Input: dimensioned drawing with shaded views. Units: mm. Origin: part minimum x, y, z. A direction names the side the tool comes from. Round coordinates to 2 decimals unless told otherwise and drop trailing zeros. Order: outer loops, then holes, each group sorted by start corner. A loop starts at its lowest first (then second) coordinate and runs counter-clockwise, first axis right, second up. Notation, with made-up numbers: M 35,-17 L 50,-17 A22 cw 50,-1 Z; hole C 0.5,67.5 d10. An arc over 180 degrees is marked long. One line per question, with ' | ' between items.
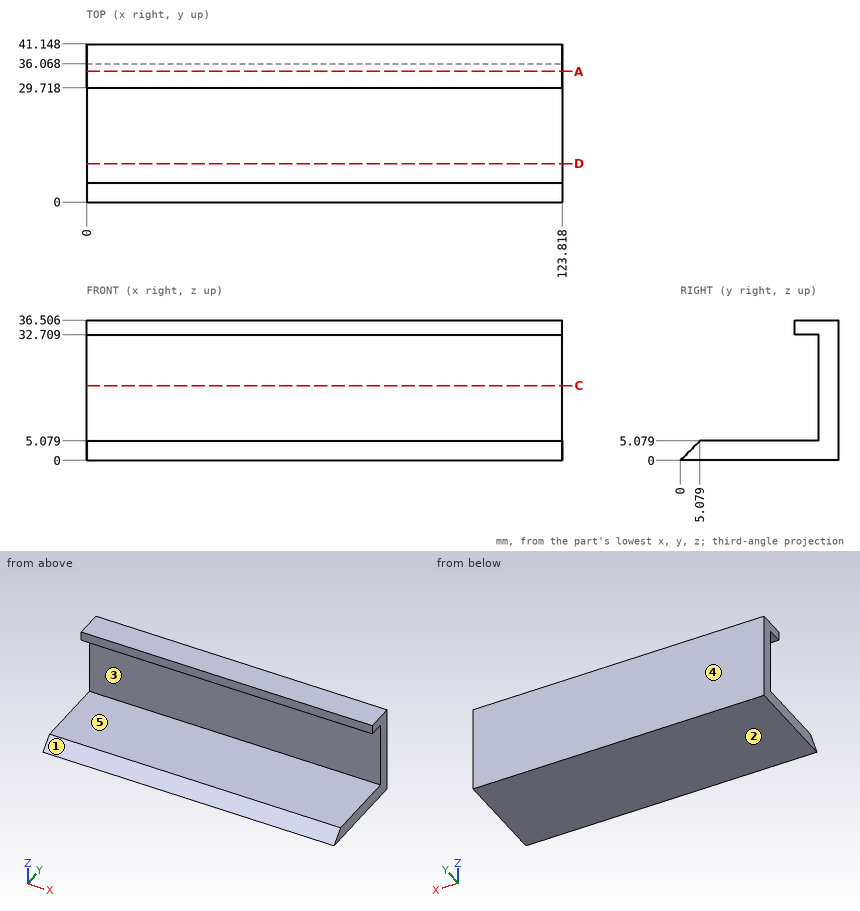
Item 1: Access query for the marked faces 4 and 5. Directions: +Z, -Z, +X, -X, +Y, -Y. A direction counts if a zero-diameter tool reaches every point of the face in a straight line with its end or side. Return the directions, or none.
Report:
face 4: +Z, -Z, +X, -X, +Y | face 5: +X, -X, -Y
Item 2: Section query A-A, the plane y = 34. Return loops of the section in (x, z).
Report:
outline: M 0,0 L 123.82,0 L 123.82,5.08 L 0,5.08 Z; M 0,32.71 L 123.82,32.71 L 123.82,36.51 L 0,36.51 Z
Item 3: Mould query, pull axis Z, two halves, no side actions, for the marked faces 1, 2 and 3. Classes: +Z half, -Z half, draft (parallel to the pull), parting line (faces both ways), or undercut.
Report:
face 1: +Z half | face 2: -Z half | face 3: undercut
Item 4: Line query: line 1 along Z through (x, y) = (72.5, 30.5); line 2 along Y through (x, z) = (17, 18); line 3 along Z through (x, y) = (99, 13). Output: solid intervals per line, ascending. Write a range as from..to.
Report:
line 1: 0..5.08, 32.71..36.51 | line 2: 36.07..41.15 | line 3: 0..5.08
Item 5: First-contact query: pin 1 (2 mm diameter, centred on x = 81.5, y = 8, fed in from +Z); pin 2 (5 mm diameter, centred on x = 81.5, z = 32.5, fed in from -Y). Flat tips, straight axial feed; report the tip coordinate or a pass-through.
Report:
pin 1: z = 5.08 | pin 2: y = 29.72
Item 6: Section query C-C, the plane z = 19.5. Return loops of the section in (x, y), plus the area to 3 significant figures.
Report:
outline: M 0,36.07 L 123.82,36.07 L 123.82,41.15 L 0,41.15 Z | area: 629 mm²
Item 7: Section query D-D, the plane y = 10. Return loops of the section in (x, z).
Report:
outline: M 0,0 L 123.82,0 L 123.82,5.08 L 0,5.08 Z
